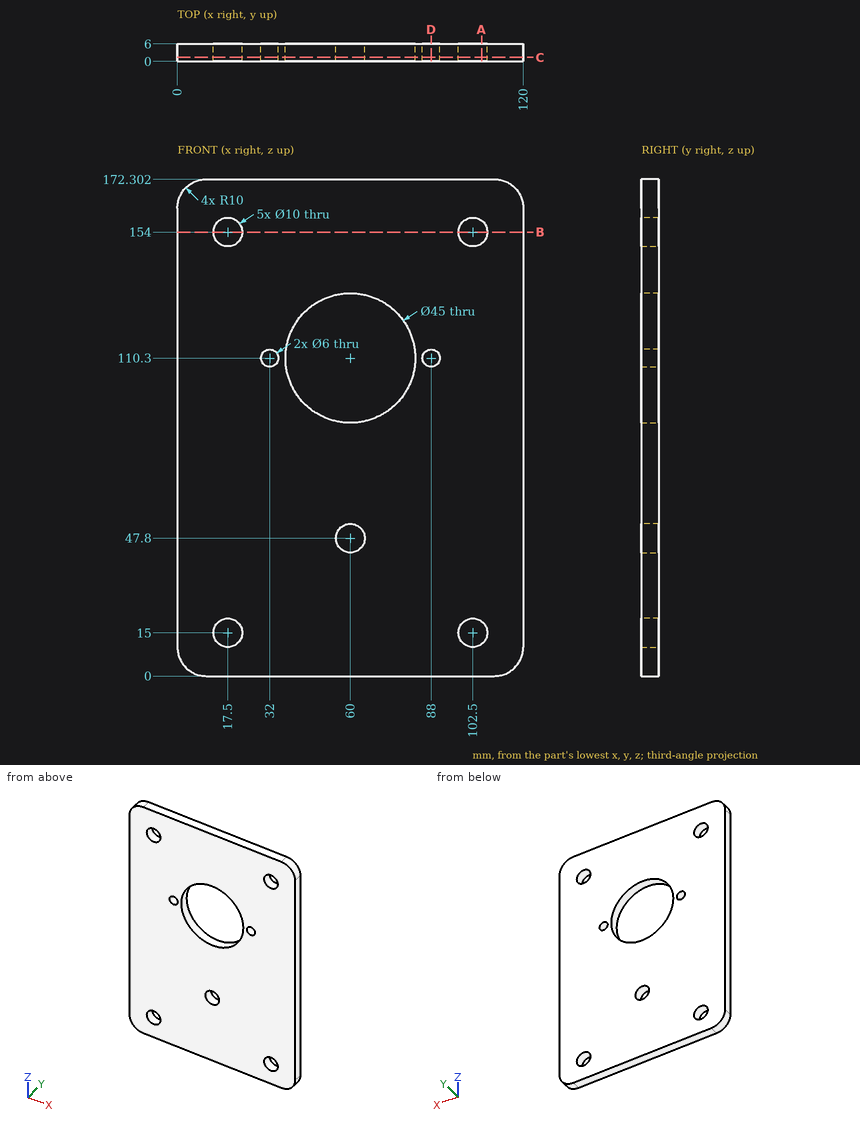
Input: dimensioned drawing with shaded views. Units: mm. Origin: part minimum x, y, z. Give positions to 0.01 mm unless a question says otherwise; leave off trailing zeros. Order: outer loops, then holes, each group sorted by start corner. A loop starts at its lowest first (then second) coordinate and runs counter-clockwise, first axis right, second up.
(1) Section query C-C (y = 1.4). State how many separate pieces and enclosed holes the cut face has, plus the area to 3 significant figures.
(2) Section query B-B (z = 154). Return the cut outline in (x, y).
(3) Section query A-A (x = 105.5). Return the cut outline in (y, z).
(4) Section query D-D (x = 88). Return the cut outline in (y, z), plus the area to 3 significant figures.
(5) Material intervals for line 1 along Z through (x, y) = (88, 2.3); line 2 along X through (y, z) = (1.7, 47.8); line 3 along X through (y, z) = (2.6, 15), sorted ascending.
Outcome:
1. separate pieces: 1
1. enclosed holes: 8
1. area: 18,600 mm2
2. outline: (0, 0) - (12.5, 0) - (12.5, 6) - (0, 6) - close; (22.5, 0) - (97.5, 0) - (97.5, 6) - (22.5, 6) - close; (107.5, 0) - (120, 0) - (120, 6) - (107.5, 6) - close
3. outline: (0, 0) - (6, 0) - (6, 11) - (0, 11) - close; (0, 19) - (6, 19) - (6, 150) - (0, 150) - close; (0, 158) - (6, 158) - (6, 172.3) - (0, 172.3) - close
4. outline: (0, 0) - (6, 0) - (6, 107.3) - (0, 107.3) - close; (0, 113.3) - (6, 113.3) - (6, 172.3) - (0, 172.3) - close
4. area: 998 mm2
5. line 1: z = 0 to 107.3, 113.3 to 172.3
5. line 2: x = 0 to 55, 65 to 120
5. line 3: x = 0 to 12.5, 22.5 to 97.5, 107.5 to 120
